from build123d import *

# Parameters (mm, degrees)
BOSS_EXTRUDE1_DEPTH = 12.7


with BuildPart() as part:
    # Sketch1 → Boss-Extrude1 (new body)
    with BuildSketch(Plane(origin=(0, 0, 0), x_dir=(0, 0, -1), z_dir=(1, 0, 0))):
        with BuildLine():
            ThreePointArc((8.586931818, -7.053528068), (-11.1125, 0), (8.586931818, 7.053528068))
            Line((8.586931818, 7.053528068), (99.363068182, 81.61939621))
            ThreePointArc((99.363068182, 81.61939621), (104.203977014, 99.134997115), (119.0625, 88.672924278))
            ThreePointArc((119.0625, 88.672924278), (118.412072837, 84.926901292), (116.536931818, 81.61939621))
            Line((116.536931818, 81.61939621), (122.670454545, 76.581161876))
            ThreePointArc((122.670454545, 76.581161876), (121.420384182, 102.14330846), (95.858237598, 103.393378823))
            Line((95.858237598, 103.393378823), (-12.091762402, 14.720454545))
            ThreePointArc((-12.091762402, 14.720454545), (-14.720454545, -12.091762402), (12.091762402, -14.720454545))
            Line((12.091762402, -14.720454545), (15.006187185, -12.326470588))
            Line((15.006187185, -12.326470588), (8.586931818, -7.053528068))
        make_face()
        with BuildLine():
            Line((99.363068182, 81.61939621), (8.586931818, 7.053528068))
            ThreePointArc((8.586931818, 7.053528068), (10.462072837, 3.746022986), (11.1125, 0))
            ThreePointArc((11.1125, 0), (10.462072837, -3.746022986), (8.586931818, -7.053528068))
            Line((8.586931818, -7.053528068), (15.006187185, -12.326470588))
            Line((15.006187185, -12.326470588), (120.041762402, 73.952469732))
            ThreePointArc((120.041762402, 73.952469732), (121.420384182, 75.202540096), (122.670454545, 76.581161876))
            Line((122.670454545, 76.581161876), (116.536931818, 81.61939621))
            ThreePointArc((116.536931818, 81.61939621), (107.95, 77.560424278), (99.363068182, 81.61939621))
        make_face()
    extrude(amount=BOSS_EXTRUDE1_DEPTH)


solid = part.part
CAD build for the part. Positions are in the model's coordinates, mm. Coordinates: 2 decimals unless noted, no trailing zeros. Write each loop counter-clockwise with the first axis right and the second up, starting at its lowest first coordinate (ties: lowest second). Pieces come first, ordered by that corner, then holes. Notation, with made-up numbers: M 35.5,-18.75 L 65.5,-18.75 A28 cw 65.5,11.25 Z; hole C -12.75,48 d9. An arc over 180 degrees is marked long. Answer as a JSON object with one key per item and string values. Group by question number.
1) Saw through at A-A (x = 11). Give the number of separate pieces and of enclosed holes in the cut face, plus the area to 3 significant figures.
2) Saw through at B-B (z = -107.95). Write the cut outline in (x, y), plus the area to 3 significant figures.
3) Wall check: line 1 (Y direction, x = 5.5, z = -107.95); line 2 (Z direction, x = 10.25, y = 6); line 3 (Z direction, x = 4, y = 0). Give the ranges that are in metal, low to high. Write a range as from..to.
4) Saw through at D-D (z = -82.5). Write the cut outline in (x, y), plus the area to 3 significant figures.
5) Pin check, flat tips, straight feed: pin 1 Ø1.5 at (x, y) = (5, 31) entering from +Z; pin 2 Ø5 at (x, y) = (8, 42) entering from +Z; pin 3 Ø1 at (x, y) = (4.5, 41) entering from -Z; pin 4 Ø5 at (y, z) = (58, -105) entering from -X. Stop position of each tip, or through.
6) Saw through at C-C (y = 17). Write the cut outline in (x, z).
Values follow:
{
 "1": {"separate pieces": "1", "enclosed holes": "2", "area": "5,690 mm2"},
 "2": {"outline": "M 0,64.02 L 12.7,64.02 L 12.7,77.56 L 0,77.56 Z; M 0,99.79 L 12.7,99.79 L 12.7,107.72 L 0,107.72 Z", "area": "273 mm2"},
 "3": {"line 1": "y = 64.02..77.56, 99.79..107.72", "line 2": "z = -37.32..-9.35, 9.35..18.08", "line 3": "z = -30.01..-11.11, 11.11..19.05"},
 "4": {"outline": "M 0,43.11 L 12.7,43.11 L 12.7,92.42 L 0,92.42 Z", "area": "626 mm2"},
 "5": {"pin 1": "stops at z = -6.81", "pin 2": "stops at z = -18.07", "pin 3": "stops at z = -80.53", "pin 4": "passes through"},
 "6": {"outline": "M 0,-50.71 L 12.7,-50.71 L 12.7,9.32 L 0,9.32 Z"}
}
